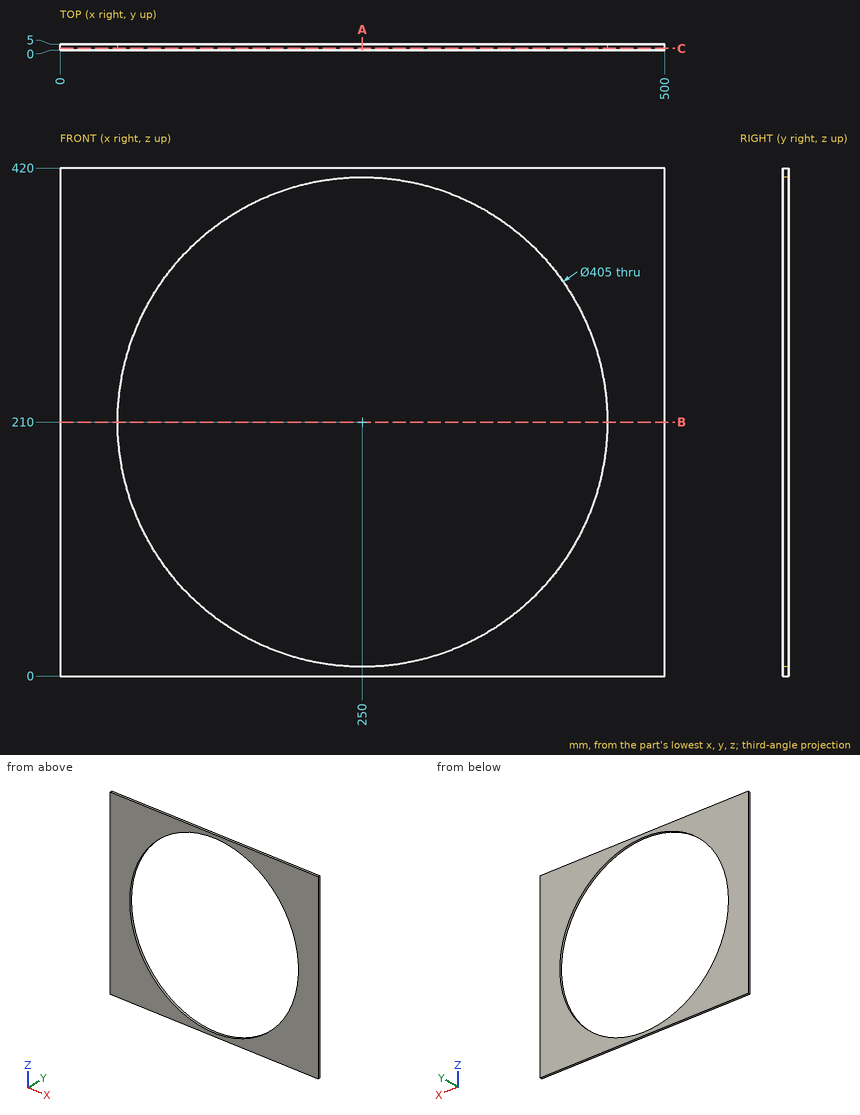
Study the drawing (mm; zero at the part's minimum x, y, z) and answer. Round coordinates to 2 decimals unless told otherwise and drop trailing zeros. Loops run counter-clockwise (first coordinate to the right, second up) from the corner with the lowest first, then second, coordinate; pieces in that order, holes last. Notation, with made-up numbers: (14.25, 34.5) -> (69.25, 34.5) arc R26 cw to (69.25, 70.5) -> close; hole circle Ø1 at (25, -31.5). An arc over 180 degrees is marked (long way). Write each question's results on one line, items separated by ' | '. Start each with the question number.
1. Find the intervals of material crossed by probe 1 along Z at (x, y) = (250, 2.75); probe 2 along X at (y, z) = (1.65, 214.5); probe 3 along X at (y, z) = (2, 227), in increasing order. Write a range as from..to.
2. Section A-A (x = 250) is taken. Determine the outline of the cut face in (y, z).
3. Section C-C (y = 1.35) is taken. Determine the outline of the cut face in (x, z), plus the area to 3 significant figures.
4. Section B-B (z = 210) is taken. Determine the outline of the cut face in (x, y).
Evaluation:
1) probe 1: z = 0..7.5, 412.5..420 | probe 2: x = 0..47.55, 452.45..500 | probe 3: x = 0..48.21, 451.79..500
2) outline: (0, 0) -> (5, 0) -> (5, 7.5) -> (0, 7.5) -> close; (0, 412.5) -> (5, 412.5) -> (5, 420) -> (0, 420) -> close
3) outline: (0, 0) -> (500, 0) -> (500, 420) -> (0, 420) -> close; hole circle Ø405 at (250, 210) | area: 81,200 mm2
4) outline: (0, 0) -> (47.5, 0) -> (47.5, 5) -> (0, 5) -> close; (452.5, 0) -> (500, 0) -> (500, 5) -> (452.5, 5) -> close
